Work out the finished part from the listing and answer in its coordinate system (mm). Face numbers are marked on the shaded views. A direction names the side the tool comes from. Give positions to 0.01 mm unless a question says otherwise; leave off trailing zeros. Loops run counter-clockwise (first coordinate to the right, second up) from the corner with the lowest first, then second, coordinate; pieces in that order, holes last. Notation, with made-up numbers: (-34, -25) - (16, -25) arc R26 cw to (16, -2) - close; hole circle Ø7 at (-8.75, 66.5). An arc over 180 degrees is marked (long way). One line per item, written item: value.
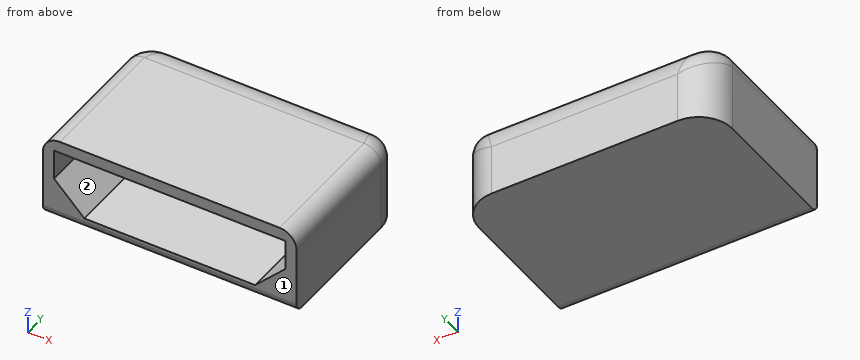
from build123d import *

# Parameters (mm, degrees)
SKETCH007_W     = 7.5
SKETCH007_H     = 5
PAD006_DEPTH    = 2.5
SKETCH008_W     = 6.85
SKETCH008_H     = 1.8
POCKET001_DEPTH = 4
FILLET_R        = 0.5
CHAMFER003_SIZE = 0.9
FILLET001_R     = 0.25
FILLET002_R     = 1


with BuildPart() as part:
    # Sketch007 (on Face1 of CopyPad003) → Pad006 (new body)
    with BuildSketch(Plane.XY.offset(1.6)):
        with Locations((0, -25.5)):
            Rectangle(SKETCH007_W, SKETCH007_H)
    extrude(amount=PAD006_DEPTH)

    # Sketch008 (on Face1 of Pad006) → Pocket001 (cut)
    with BuildSketch(Plane(origin=(0, -28, 1.6), x_dir=(1, 0, 0), z_dir=(0, -1, 0))):
        with Locations((0, 1.25)):
            Rectangle(SKETCH008_W, SKETCH008_H)
    extrude(amount=-POCKET001_DEPTH, mode=Mode.SUBTRACT)

    # Fillet
    fillet_edges = [part.edges().sort_by_distance(p)[0] for p in [
        (-3.75, -25.5, 4.1),
        (3.75, -25.5, 4.1),
    ]]
    fillet(fillet_edges, radius=FILLET_R)

    # Chamfer003
    chamfer003_edges = [part.edges().sort_by_distance(p)[0] for p in [
        (3.425, -26, 1.95),
        (-3.425, -26, 1.95),
    ]]
    chamfer(chamfer003_edges, length=CHAMFER003_SIZE)

    # Fillet001
    fillet001_edges = [part.edges().sort_by_distance(p)[0] for p in [
        (0, -28, 1.6),
    ]]
    fillet(fillet001_edges, radius=FILLET001_R)

    # Fillet002
    fillet002_edges = [part.edges().sort_by_distance(p)[0] for p in [
        (0, -23, 4.1),
    ]]
    fillet(fillet002_edges, radius=FILLET002_R)


with BuildPart() as part_1:
    # Body006 placement: moved
    add(part.part.moved(Location((0, 3, 0))))


solid = part_1.part
1. Find the intervals of material crossed by line 1 along Z through (x, y) = (1.25, -21.8); line 2 along X through (y, z) = (-24.5, 3.55) (3 decimals); line 3 along Y through (x, z) = (-1.25, 2.65), in increasing order.
Output:
line 1: z = 1.6 to 1.95, 3.75 to 4.1
line 2: x = -3.75 to -3.425, 3.425 to 3.75
line 3: y = -21 to -20
2. Section B-B (z = 2.95) is taken. Write down the section's boundary in (x, y) (3 decimals), and give its area (3 significant figures).
Output:
outline: (-3.75, -25) - (-3.425, -25) - (-3.425, -21) - (3.425, -21) - (3.425, -25) - (3.75, -25) - (3.75, -21) arc R1 ccw to (2.75, -20) - (-2.75, -20) arc R1 ccw to (-3.75, -21) - close
area: 9.67 mm²
3. Section A-A (y = -23.1) is taken. Write down the section's boundary in (x, z) (3 decimals), and give its area (3 significant figures).
Output:
outline: (-3.75, 1.6) - (3.75, 1.6) - (3.75, 3.6) arc R0.5 ccw to (3.25, 4.1) - (-3.25, 4.1) arc R0.5 ccw to (-3.75, 3.6) - close; hole (-3.425, 2.85) - (-2.525, 1.95) - (2.525, 1.95) - (3.425, 2.85) - (3.425, 3.75) - (-3.425, 3.75) - close
area: 7.12 mm²
4. For the marked faces 1 and 2, determine the directions among +Z, -Z, +X, -X, +Y, -Y from which every point of the face is accessible in a straight line to the end or side of a thin tool.
Output:
face 1: +Z, -Z, +X, -X, -Y
face 2: -Y
5. Section C-C (x = 0.5) is taken. Write down the section's boundary in (y, z).
Output:
outline: (-25, 1.85) arc R0.25 ccw to (-24.75, 1.6) - (-20, 1.6) - (-20, 3.1) arc R1 ccw to (-21, 4.1) - (-25, 4.1) - (-25, 3.75) - (-21, 3.75) - (-21, 1.95) - (-25, 1.95) - close
